Model file for the job. Use its own axes, mm. Face numbers are marked on the shaded views. Coordinates: 2 decimals unless noted, no trailing zeros. Write each loop counter-clockwise with the first axis right and the second up, starting at its lowest first coordinate (ties: lowest second). Pieces come first, ordered by that corner, then holes. Notation, with made-up numbers: M 9.25,59 L 50.25,59 A12 cw 50.25,67 Z; hole C 53,-25 d5. An arc over 180 degrees is marked long. Put each result on its own line as item: value. Start each with the question number.
Q1. Pull direction X, two halves, no side cores. Call the marked faces 1, 2 and 3: pulls with the +X half, pulls with the -X half, needs draft (parallel to the pull), parting line crosses it, or undercut.
Q2. Drop a flat-ended pin along its axis: pin 1 (5 mm diameter, centred on x = -27.5, z = -9, fed in from -Y). Give the stop position or say it passes through.
Q3. Drill centre lines: line 1 along X through (y, z) = (10.25, 0); line 2 along Z through (x, y) = (22.5, 15.25); line 3 along Z through (x, y) = (0, 11). Where is each one in solid material? Low to high.
Q4. Cut at D-D (x = -22.5). Write the cut outline in (y, z).
Q5. Cut at C-C (y = 4.75). Write the cut outline in (x, z).
Q6. Cut at A-A (z = 0). Write the cut outline in (x, y).
Q7. Cut at B-B (x = 22.5). Write the cut outline in (y, z), then the cut area to 3 significant figures.
Autodesk Inventor part; units mm, degrees
ref_plane "YZ Plane" through (0, 0, 0) normal (1, 0, 0) x (0, 1, 0)
ref_plane "XZ Plane" through (0, 0, 0) normal (0, 1, 0) x (-1, 0, 0)
ref_plane "XY Plane" through (0, 0, 0) normal (0, 0, 1) x (1, 0, 0)
sketch "Boceto1" plane through (0, 0, 0) normal (0, 1, 0) x (-1, 0, 0)
  line L0 (45, 22.5) -> (-45, 22.5)
  line L1 (-45, 22.5) -> (-45, -22.5)
  line L2 (-45, -22.5) -> (45, -22.5)
  line L3 (45, -22.5) -> (45, 22.5)
  point P0 (-45, 0)
extrude "Extrusión1" add sketch "Boceto1" along normal blind 24
sketch "Boceto2" plane through (0, 24, 0) normal (0, 1, 0) x (1, 0, 0)
  point P0 (-22.5, 0)
hole "Agujero1" at (-22.5, 24, 0) direction (0, -1, 0) diameter 7.5 end through all countersink diameter 12 countersink angle 90
sketch "Boceto3" plane through (0, 24, 0) normal (0, 1, 0) x (1, 0, 0)
  point P0 (0, 0)
hole "Agujero2" at (0, 24, 0) direction (0, -1, 0) diameter 12 end through all countersink diameter 16 countersink angle 82
sketch "Boceto4" plane through (0, 24, 0) normal (0, 1, 0) x (1, 0, 0)
  point P0 (0, 0)
  point P1 (0, 0)
  point P2 (22.5, 0)
hole "Agujero3" at (0, 24, 0) at (22.5, 24, 0) direction (0, -1, 0) diameter 7.5 end through all countersink diameter 12 countersink angle 82
properties part number "sujecion_castor" material "Aluminio 6061"
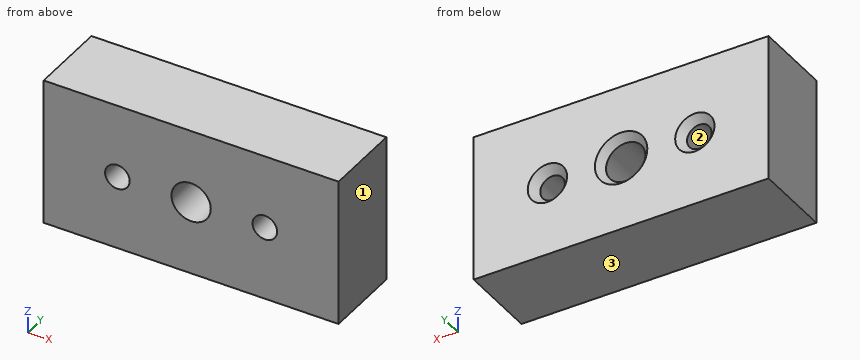
Computed values:
1. face 1: pulls with the +X half
1. face 2: undercut
1. face 3: needs draft
2. pin 1: y = 0
3. line 1: -45 to -26.25, -18.75 to -6, 6 to 18.75, 26.25 to 45
3. line 2: -22.5 to -3.75, 3.75 to 22.5
3. line 3: -22.5 to -6, 6 to 22.5
4. outline: M 0,-22.5 L 24,-22.5 L 24,-6 L 21.75,-3.75 L 0,-3.75 Z; M 0,3.75 L 21.75,3.75 L 24,6 L 24,22.5 L 0,22.5 Z
5. outline: M -45,-22.5 L 45,-22.5 L 45,22.5 L -45,22.5 Z; hole C -22.5,0 d7.5; hole C 0,0 d12; hole C 22.5,0 d7.5
6. outline: M -45,0 L -26.25,0 L -26.25,21.75 L -28.5,24 L -45,24 Z; M -18.75,0 L -6,0 L -6,21.7 L -8,24 L -16.5,24 L -18.75,21.75 Z; M 6,0 L 18.75,0 L 18.75,21.41 L 16.5,24 L 8,24 L 6,21.7 Z; M 26.25,0 L 45,0 L 45,24 L 28.5,24 L 26.25,21.41 Z
7. outline: M 0,-22.5 L 24,-22.5 L 24,-6 L 21.41,-3.75 L 0,-3.75 Z; M 0,3.75 L 21.41,3.75 L 24,6 L 24,22.5 L 0,22.5 Z
7. area: 894 mm2
